Verification items for the finished model (mm, model axes). Face numbers are marked on the shaded views. A direction names the side the tool comes from. Coordinates: 2 decimals unless noted, no trailing zeros. Write each loop counter-clockwise with the first axis right and the second up, starting at its lowest first coordinate (ties: lowest second). Pieces come first, ordered by that corner, then holes. Notation, with made-up numbers: (74, -14) -> (81, -14) arc R23 cw to (81, 16) -> close; hole circle Ø9 at (15.5, -22.5). An arc over 180 degrees is marked (long way). Use CSV: the item, a comma, the result in double quotes.
```python
from build123d import *

# Parameters (mm, degrees)
F0_W     = 16.6666666667
F0_H     = 50
F0_W_2   = 48.3333333333
F2_R     = 7.5
F3_SIZE  = 5
F4_SIZE2 = 5
F4_SIZE  = 3.8


with BuildPart() as f1:
    # F0 (on Right) → F1 (revolve)
    with BuildSketch(Plane.YZ):
        with Locations((8.3333333333, 100)):
            Rectangle(F0_W, F0_H)
        with Locations((8.3333333333, 50)):
            Rectangle(F0_W, F0_H)
        with Locations((40.8333333333, 50)):
            Rectangle(F0_W_2, F0_H)
    revolve(axis=Axis((0, 32.5, 0), (0, 1, 0)))

    # F2
    f2_edges = [f1.edges().sort_by_distance(p)[0] for p in [
        (0, 16.666667, -75),
    ]]
    fillet(f2_edges, radius=F2_R)

    # F3
    f3_edges = [f1.edges().sort_by_distance(p)[0] for p in [
        (0, 65, -75),
    ]]
    chamfer(f3_edges, length=F3_SIZE)

    # F4
    f4_edges = [f1.edges().sort_by_distance(p)[0] for p in [
        (0, 0, -125),
        (0, 16.666667, -125),
    ]]
    f4_side = f1.faces().sort_by_distance((0, 8.333333, -125))[0]
    chamfer(f4_edges, length=F4_SIZE, length2=F4_SIZE2, reference=f4_side)


solid = f1.part
```
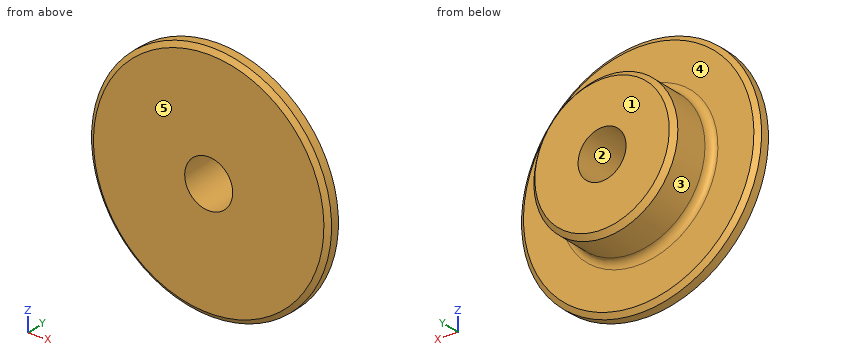
1) Cross-section at A-A (x = 0). Record the boundary of the cut face in (y, z).
Return value:
outline,"(0, -120) -> (3.8, -125) -> (12.87, -125) -> (16.67, -120) -> (16.67, -82.5) arc R7.5 cw to (24.17, -75) -> (60, -75) -> (65, -70) -> (65, -25) -> (0, -25) -> close; (0, 25) -> (65, 25) -> (65, 70) -> (60, 75) -> (24.17, 75) arc R7.5 cw to (16.67, 82.5) -> (16.67, 120) -> (12.87, 125) -> (3.8, 125) -> (0, 120) -> close"
2) Set-up check for the marked faces 4 and 5: record each of +Z, -Z, +X, -X, +Y, -Y from which the full face is reachable in a straight line by a thin tool's end or side.
Return value:
face 4,"+Y"
face 5,"+Z, -Z, +X, -X, -Y"
3) Mould release check, pull along Z, two halves, no side actions. Record for the marked faces 1, 2 and 3: released by +Z, released by -Z, zero draft, split by the parting line, or undercut.
Return value:
face 1,"zero draft"
face 2,"undercut"
face 3,"split by the parting line"
4) Scan lines: L1, parallel to X at y = 39, z = 0; L2, parallel to Y at x = -48.5, z = 105; L3, parallel to X at y = 19, z = 0. Record each from-to range of solid material in increasing order.
Return value:
L1,"-75 to -25, 25 to 75"
L2,"0 to 16.67"
L3,"-77.06 to -25, 25 to 77.06"
5) Cross-section at B-B (z = 0). Record the boundary of the cut face in (x, y).
Return value:
outline,"(-125, 3.8) -> (-120, 0) -> (-25, 0) -> (-25, 65) -> (-70, 65) -> (-75, 60) -> (-75, 24.17) arc R7.5 cw to (-82.5, 16.67) -> (-120, 16.67) -> (-125, 12.87) -> close; (25, 0) -> (120, 0) -> (125, 3.8) -> (125, 12.87) -> (120, 16.67) -> (82.5, 16.67) arc R7.5 cw to (75, 24.17) -> (75, 60) -> (70, 65) -> (25, 65) -> close"
6) Gauge pin test, flat ends, axial feed: pin 1 (1.5 mm diameter, centred on y = 53.5, z = 67, fed in from +X); pin 2 (4 mm diameter, centred on y = 29, z = -63, fed in from +X); pin 3 (4 mm diameter, centred on x = -28, z = -85, fed in from +Y). Record the tip position at first contact, or that the pin passes through.
Return value:
pin 1,"x = 35.16"
pin 2,"x = 43.63"
pin 3,"y = 16.67"
7) Cross-section at C-C (y = 46.5). Record the boundary of the cut face in (x, z).
Return value:
outline,"circle Ø150 at (0, 0); hole circle Ø50 at (0, 0)"
